Here's the drawing with two shaded views (mm, measured from the low corner). I have some questions. A direction names the side the tool comes from. Round coordinates to 2 decimals unless told otherwise and drop trailing zeros. Loops run counter-clockwise (first coordinate to the right, second up) from the corner with the lowest first, then second, coordinate; pieces in that order, holes last. Notation, with made-up numbers: (-14, 87.25) -> (32, 87.25) arc R12 cw to (32, 91.25) -> close; hole circle Ø6 at (34.5, -32). An arc over 180 degrees is marked (long way). Write each question's results on one line, items separated by ' | '. Start each with the question number.
1) Imagine slicing it at A-A, the plane z = 15. List the corners of the cut face in (x, y) for me, plus the area to 3 significant figures.
2) If I drill on probe 1 along Z at (x, y) = (15, 46); probe 2 along Y at (x, z) = (15.5, 18.5); probe 3 along Y at (x, z) = (8, 17), over which ranges is the centre line in solid material (lowest first)?
3) For P1, Ø1, axis at x = 20.5, y = 22.5, coming from the +Z side; P2, Ø4, axis at y = 21.5, z = 20, coming from the +X side; P3, Ø1, axis at x = 25, y = 38.5, coming from the -Z side, each with a flat end and sliding along its axis, tell me the tip position at first contact or that it passes through.
4) Imagine slicing it at D-D, the plane y = 9. List the corners of the cut face in (x, z) for me, plus the area to 3 significant figures.
5) Imagine slicing it at B-B, the plane x = 15. List the corners of the cut face in (y, z) for me.
6) We'd pull the mould along Z, two halves only. Please class the marked faces 3, 4 and 5: pulls with the +Z half, pulls with the -Z half, needs draft (parallel to the pull), parting line crosses it, or undercut.
7) Which directions (+Z, -Z, +X, -X, +Y, -Y) give clear straight access to the entire face, cutting with the end or side of a thin tool? Please do the marked faces 1 and 2.
8) Imagine slicing it at C-C, the plane y = 46. List the corners of the cut face in (x, z) for me, plus the area to 3 significant figures.
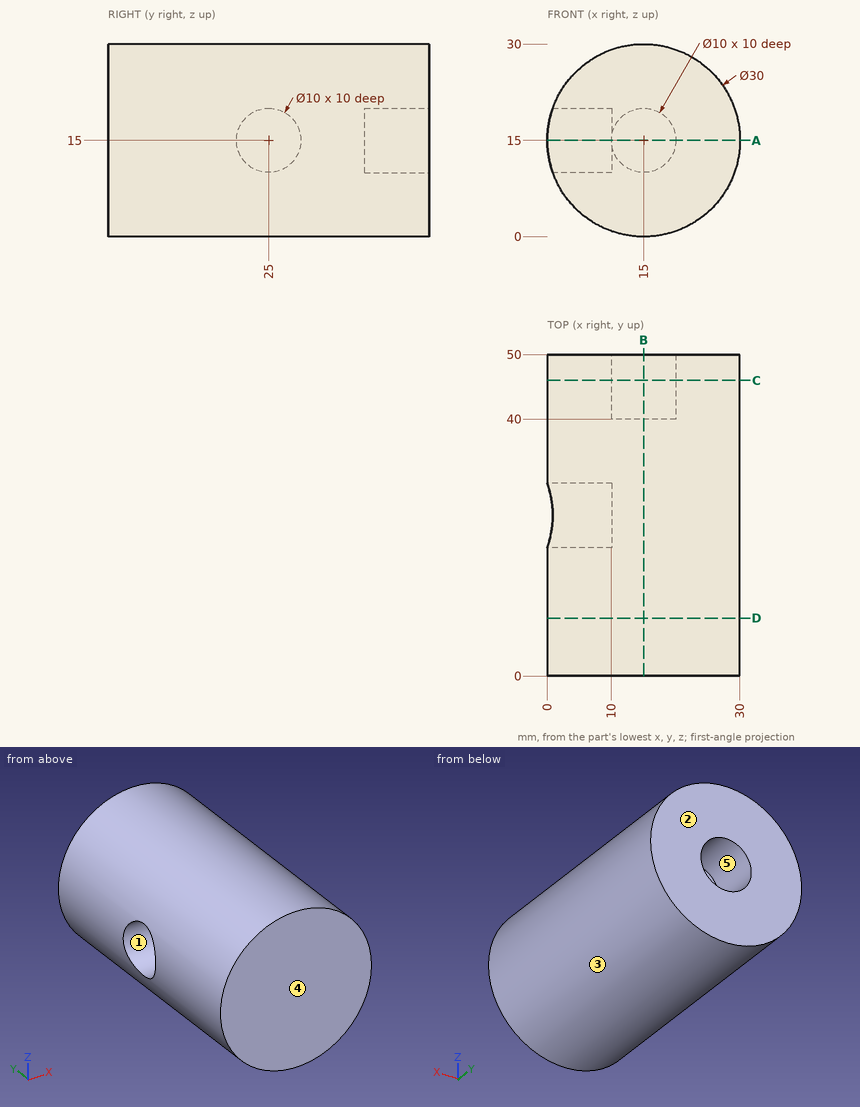
Checked values:
1) outline: (0, 0) -> (30, 0) -> (30, 50) -> (20, 50) -> (20, 40) -> (10, 40) -> (10, 50) -> (0, 50) -> (0, 30) -> (10, 30) -> (10, 20) -> (0, 20) -> close | area: 1,300 mm^2
2) probe 1: 0 to 10, 20 to 30 | probe 2: 0 to 40 | probe 3: 0 to 20.42, 29.58 to 50
3) P1: z = 29.14 | P2: x = 29.7 | P3: z = 3.39
4) outline: circle Ø30 at (15, 15) | area: 707 mm^2
5) outline: (0, 0) -> (50, 0) -> (50, 10) -> (40, 10) -> (40, 20) -> (50, 20) -> (50, 30) -> (0, 30) -> close
6) face 3: parting line crosses it | face 4: needs draft | face 5: undercut
7) face 1: -X | face 2: +Z, -Z, +X, -X, +Y
8) outline: circle Ø30 at (15, 15); hole circle Ø10 at (15, 15) | area: 628 mm^2
